For this review, take the finished solid that the model builds, in its own axes (mm). Face numbers are marked on the shaded views. A direction names the side the tool comes from. Give positions to 0.01 mm unless a question says otherwise; leave off trailing zeros. Write each loop counter-clockwise with the first axis right and the second up, starting at its lowest first coordinate (ties: lowest second). Pieces come first, ordered by that corner, then holes.
1) For P1, Ø3.5, axis at x = -53.5, y = 36.5, coming from the +Z side; P2, Ø1.5, axis at x = -53.5, y = 36, coming from the -Z side; P3, Ø1.5, axis at x = 52, y = 36, coming from the +Z side, all flat-tipped, find the tip position at first contact; note any pin that passes through.
2) Draft analysis for pull direction Z (two halves, no side actions). For the marked faces 3, 4 and 5, state which applies: pulls with the +Z half, pulls with the -Z half, needs draft (parallel to the pull), parting line crosses it, or undercut.
3) Wall thickness on line 1 along Z through (x, y) = (-44, 23.5); line 2 along X through (y, z) = (32, 47); line 3 along Y through (x, z) = (-29, 31): over which ranges is each line inside the solid? List them lowest first.
4) We need section C-C on z = 80.5. Give the boundary of the cut face in (x, y), and give its area (3 significant figures).
5) We need section D-D on y = 17. Give the boundary of the cut face in (x, z).
6) We need section A-A on x = 24.5. Give the boundary of the cut face in (y, z).
7) We need section B-B on y = 30. Give the boundary of the cut face in (x, z).
8) Machinability: for the marked faces 1 and 2, which of the approach directions +Z, -Z, +X, -X, +Y, -Y give a long, thin tool a straight path to every point of the face, cutting with its end or side? Answer none if there is none.
from build123d import *

# Parameters (mm, degrees)
SKETCH1_W           = 109.3
SKETCH1_H           = 100
BOSS_EXTRUDE1_DEPTH = 35
SKETCH2_W           = 2.5
SKETCH2_H           = 7
BOSS_EXTRUDE2_DEPTH = 3
SKETCH3_W           = 7
SKETCH3_H           = 1
BOSS_EXTRUDE3_DEPTH = 1
SKETCH4_W           = 7
SKETCH4_H           = 1
BOSS_EXTRUDE4_DEPTH = 1
FILLET1_R           = 0.5
SKETCH5_W           = 105.3
SKETCH5_H           = 96
CUT_EXTRUDE1_DEPTH  = 33
FILLET2_R           = 5
SKETCH6_W           = 1
SKETCH6_H           = 3
CUT_EXTRUDE2_DEPTH  = 153.939497841
CUT_EXTRUDE3_REACH  = 122.128
SKETCH7_W           = 80
SKETCH7_H           = 14


with BuildPart() as part:
    # Sketch1 → Boss-Extrude1 (new body)
    with BuildSketch(Plane(origin=(0, 0, 0), x_dir=(1, 0, 0), z_dir=(0, 1, 0))):
        with Locations((0, -50)):
            Rectangle(SKETCH1_W, SKETCH1_H)
    extrude(amount=BOSS_EXTRUDE1_DEPTH)

    # Sketch2 → Boss-Extrude2 (add)
    with BuildSketch(Plane(origin=(0, 35, 0), x_dir=(1, 0, 0), z_dir=(0, 1, 0))):
        with Locations((-53.4, -13.5)):
            Rectangle(SKETCH2_W, SKETCH2_H)
        with Locations((53.4, -13.5)):
            Rectangle(SKETCH2_W, SKETCH2_H)
        with Locations((53.4, -64.52)):
            Rectangle(SKETCH2_W, SKETCH2_H)
        with Locations((-53.4, -64.52)):
            Rectangle(SKETCH2_W, SKETCH2_H)
    extrude(amount=BOSS_EXTRUDE2_DEPTH)

    # Sketch3 → Boss-Extrude3 (add)
    with BuildSketch(Plane(origin=(-52.15, 0, 0), x_dir=(0, 0, -1), z_dir=(1, 0, 0))):
        with Locations((-13.5, 37.5)):
            Rectangle(SKETCH3_W, SKETCH3_H)
        with Locations((-64.52, 37.5)):
            Rectangle(SKETCH3_W, SKETCH3_H)
    extrude(amount=BOSS_EXTRUDE3_DEPTH)

    # Sketch4 → Boss-Extrude4 (add)
    with BuildSketch(Plane.ZY.offset(-52.15)):
        with Locations((13.5, 37.5)):
            Rectangle(SKETCH4_W, SKETCH4_H)
        with Locations((64.52, 37.5)):
            Rectangle(SKETCH4_W, SKETCH4_H)
    extrude(amount=BOSS_EXTRUDE4_DEPTH)

    # Fillet1
    fillet1_edges = [part.edges().sort_by_distance(p)[0] for p in [
        (51.15, 38, 13.5),
        (51.15, 37, 13.5),
        (51.15, 37, 64.52),
        (51.15, 38, 64.52),
        (-51.15, 37, 13.5),
        (-51.15, 38, 13.5),
        (-51.15, 37, 64.52),
        (-51.15, 38, 64.52),
    ]]
    fillet(fillet1_edges, radius=FILLET1_R - 0.0001)  # a hair under: the kernel refuses the full size

    # Sketch5 → Cut-Extrude1 (cut)
    with BuildSketch(Plane(origin=(0, 35, 0), x_dir=(1, 0, 0), z_dir=(0, 1, 0))):
        with Locations((0, -50)):
            Rectangle(SKETCH5_W, SKETCH5_H)
    extrude(amount=-CUT_EXTRUDE1_DEPTH, mode=Mode.SUBTRACT)

    # Fillet2
    fillet2_edges = [part.edges().sort_by_distance(p)[0] for p in [
        (-52.65, 18.5, 98),
        (-52.65, 18.5, 2),
        (52.65, 18.5, 2),
        (52.65, 18.5, 98),
        (-54.65, 17.5, 0),
        (54.65, 17.5, 0),
        (54.65, 17.5, 100),
        (-54.65, 17.5, 100),
    ]]
    fillet(fillet2_edges, radius=FILLET2_R)

    # Sketch6 → Cut-Extrude2 (cut, through all)
    with BuildSketch(Plane.ZY.offset(54.65)):
        with Locations((10.5, 36.5)):
            Rectangle(SKETCH6_W, SKETCH6_H)
        with Locations((16.5, 36.5)):
            Rectangle(SKETCH6_W, SKETCH6_H)
        with Locations((61.52, 36.5)):
            Rectangle(SKETCH6_W, SKETCH6_H)
        with Locations((67.52, 36.5)):
            Rectangle(SKETCH6_W, SKETCH6_H)
    extrude(amount=-CUT_EXTRUDE2_DEPTH, mode=Mode.SUBTRACT)

    # Sketch7 → Cut-Extrude3 (cut, up to next)
    with BuildSketch(Plane(origin=(0, 0, 0), x_dir=(-1, 0, 0), z_dir=(0, 0, -1)), mode=Mode.PRIVATE) as cut_extrude3_sk1:
        with Locations((0, 11.66099816)):
            Rectangle(SKETCH7_W, SKETCH7_H)
    cut_extrude3_tool1 = extrude(cut_extrude3_sk1.sketch, amount=-CUT_EXTRUDE3_REACH, mode=Mode.PRIVATE) & part.part
    add(cut_extrude3_tool1.solids().sort_by_distance((0, 11.660998, 0))[0], mode=Mode.SUBTRACT)


solid = part.part
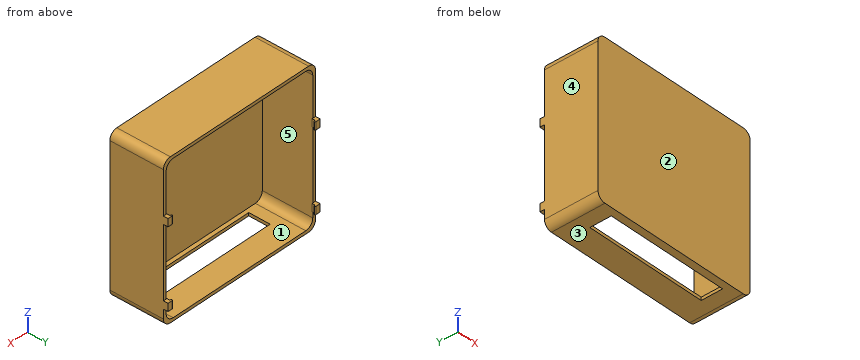
Results list:
1. P1: stops at z = 99.04
1. P2: stops at z = 11
1. P3: stops at z = 67.02
2. face 3: pulls with the -Z half
2. face 4: needs draft
2. face 5: undercut
3. line 1: z = 0 to 2, 98 to 100
3. line 2: x = -54.65 to -52.65, 52.65 to 54.65
3. line 3: y = 0 to 2
4. outline: (-54.65, 0) - (54.65, 0) - (54.65, 35) - (52.65, 35) - (52.65, 2) - (-52.65, 2) - (-52.65, 35) - (-54.65, 35) - close
4. area: 351 mm2
5. outline: (-54.65, 5) arc R5 ccw to (-49.65, 0) - (-40, 0) - (-40, 2) - (-47.65, 2) arc R5 cw to (-52.65, 7) - (-52.65, 93) arc R5 cw to (-47.65, 98) - (47.65, 98) arc R5 cw to (52.65, 93) - (52.65, 7) arc R5 cw to (47.65, 2) - (40, 2) - (40, 0) - (49.65, 0) arc R5 ccw to (54.65, 5) - (54.65, 95) arc R5 ccw to (49.65, 100) - (-49.65, 100) arc R5 ccw to (-54.65, 95) - close
6. outline: (0, 0) - (4.66, 0) - (4.66, 2) - (2, 2) - (2, 98) - (35, 98) - (35, 100) - (0, 100) - close; (18.66, 0) - (35, 0) - (35, 2) - (18.66, 2) - close
7. outline: (-54.65, 5) arc R5 ccw to (-49.65, 0) - (49.65, 0) arc R5 ccw to (54.65, 5) - (54.65, 95) arc R5 ccw to (49.65, 100) - (-49.65, 100) arc R5 ccw to (-54.65, 95) - close; hole (-52.65, 7) arc R5 ccw to (-47.65, 2) - (47.65, 2) arc R5 ccw to (52.65, 7) - (52.65, 93) arc R5 ccw to (47.65, 98) - (-47.65, 98) arc R5 ccw to (-52.65, 93) - close
8. face 1: +Y
8. face 2: +Z, -Z, +X, -X, -Y
